CAD build for the part. Positions are in the model's coordinates, mm. Face numbers are marked on the shaded views. A direction names the side the tool comes from. Give positions to 0.01 mm unless a question says otherwise; leave off trailing zeros. Loops run counter-clockwise (first coordinate to the right, second up) from the corner with the lowest first, then second, coordinate; pieces in that order, holes last. Notation, with made-up numbers: M 50.5,41.25 L 99.5,41.25 A16 ccw 99.5,57.25 Z; hole C 53.5,16 d2. An arc over 180 degrees is marked long. Answer as CSV lines item,"result".
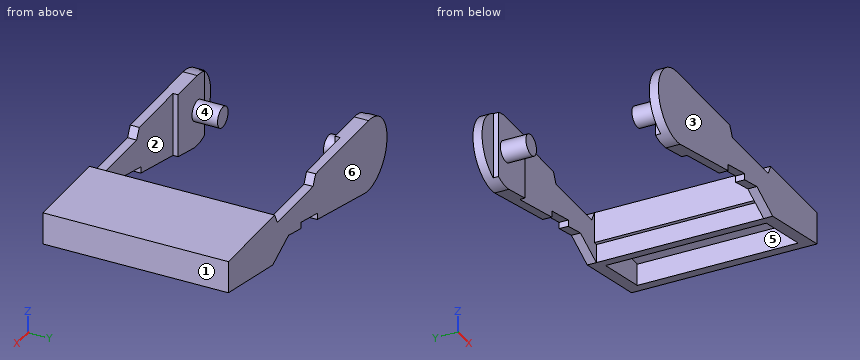
from build123d import *

# Parameters (mm, degrees)
CYLINDER_R        = 0.8
CYLINDER_DEPTH    = 2
CYLINDER001_R     = 0.8
CYLINDER001_DEPTH = 2
BOX004_W          = 0.3
BOX004_H          = 12.95
BOX004_DEPTH      = 3.2
BOX003_W          = 4.8
BOX003_H          = 12.45
BOX003_DEPTH      = 4.6
BOX001_W          = 1.7
BOX001_H          = 12.95
BOX001_DEPTH      = 10
BOX002_W          = 11.3
BOX002_H          = 12.95
BOX002_DEPTH      = 10
BOX_W             = 15.8
BOX_H             = 12.15
BOX_DEPTH         = 10
EXTRUDE_DEPTH     = 14.35


with BuildPart() as cylinder:
    # Cylinder → Cylinder (new body)
    with BuildSketch(Plane(origin=(2.8, -4.1, 2.8), x_dir=(1, 0, 0), z_dir=(0, -1, 0))):
        Circle(CYLINDER_R)
    extrude(amount=CYLINDER_DEPTH)


with BuildPart() as cylinder001:
    # Cylinder001 → Cylinder001 (new body)
    with BuildSketch(Plane(origin=(2.8, 6.1, 2.8), x_dir=(1, 0, 0), z_dir=(0, -1, 0))):
        Circle(CYLINDER001_R)
    extrude(amount=CYLINDER001_DEPTH)


with BuildPart() as cube004:
    # Box004 → Box004 (new body)
    with BuildSketch(Plane(origin=(17, -6.475, 0), x_dir=(1, 0, 0), z_dir=(0, 0, 1))):
        with Locations((0.15, 6.475)):
            Rectangle(BOX004_W, BOX004_H)
    extrude(amount=BOX004_DEPTH)


with BuildPart() as compound001:
    # Box003 → Box003 (new body)
    with BuildSketch(Plane(origin=(18.2, -6.225, 0), x_dir=(1, 0, 0), z_dir=(0, 0, 1))):
        with Locations((2.4, 6.225)):
            Rectangle(BOX003_W, BOX003_H)
    extrude(amount=BOX003_DEPTH)

    # Compound001: union Cube004
    add(cube004.part)


with BuildPart() as cube001:
    # Box001 → Box001 (new body)
    with BuildSketch(Plane(origin=(0, -6.475, 0), x_dir=(1, 0, 0), z_dir=(0, 0, 1))):
        with Locations((0.85, 6.475)):
            Rectangle(BOX001_W, BOX001_H)
    extrude(amount=BOX001_DEPTH)


with BuildPart() as compound:
    # Box002 → Box002 (new body)
    with BuildSketch(Plane(origin=(5.7, -6.475, 0), x_dir=(1, 0, 0), z_dir=(0, 0, 1))):
        with Locations((5.65, 6.475)):
            Rectangle(BOX002_W, BOX002_H)
    extrude(amount=BOX002_DEPTH)

    # Compound: union Cube001
    add(cube001.part)


with BuildPart() as cube:
    # Box → Box (new body)
    with BuildSketch(Plane(origin=(0, -6.075, 0), x_dir=(1, 0, 0), z_dir=(0, 0, 1))):
        with Locations((7.9, 6.075)):
            Rectangle(BOX_W, BOX_H)
    extrude(amount=BOX_DEPTH)


with BuildPart() as fusion:
    # Sketch → Extrude (new body)
    with BuildSketch(Plane.XZ):
        with BuildLine():
            ThreePointArc((2.8, 5.6), (0.010655, 2.555964), (3.286215, 0.042538))
            Line((3.286215, 0.042538), (10.556406, 1.8))
            Line((10.556406, 1.8), (10.556406, 2.3))
            Line((10.556406, 2.3), (13.056406, 2.904338))
            Line((13.056406, 2.404338), (13.056406, 2.904338))
            Line((13.056406, 2.404338), (14.9, 2.85))
            Line((14.9, 2.85), (17.3, 1.75))
            Line((17.3, 1.75), (24, 3.1))
            Line((24, 5.6), (24, 3.1))
            Line((17, 5.6), (24, 5.6))
            Line((16.6, 4.8), (17, 5.6))
            Line((11.2, 4.8), (16.6, 4.8))
            Line((11.2, 4.8), (10.8, 5.6))
            Line((2.8, 5.6), (10.8, 5.6))
        make_face()
    extrude(amount=EXTRUDE_DEPTH)


with BuildPart() as fusion_1:
    # Extrude placement: moved
    add(fusion.part.moved(Location((0, 7.175, 0))))

    # Cut: cut Cube
    add(cube.part, mode=Mode.SUBTRACT)

    # Cut001: cut Compound
    add(compound.part, mode=Mode.SUBTRACT)

    # Cut002: cut Compound001
    add(compound001.part, mode=Mode.SUBTRACT)

    # Fusion: union Cylinder, Cylinder001
    add(cylinder.part)
    add(cylinder001.part)


solid = fusion_1.part
1) Which spindle directions (+Z, -Z, +X, -X, +Y, -Y) get a long thin tool onto all of the face, cutting with end or side? Do the marked faces 4, 5 and 6. Say none if no direction does.
Answer below:
face 4,"none"
face 5,"-Z"
face 6,"+Z, -Z, +X, -X, +Y"
2) Drill centre lines: line 1 (Y direction, x = 14.25, z = 3.4) (3 decimals); line 2 (Y direction, x = 18.25, z = 3.95) (3 decimals); line 3 (X direction, y = 4.5, z = 4.2). Where is each one in solid material? Low to high. Write a range as from..to.
Answer below:
line 1,"y = -7.175..-6.475, 6.475..7.175"
line 2,"y = -7.175..-6.225, 6.225..7.175"
line 3,"x = 17..18.2, 23..24"
3) Flat gauge pins, fed straight in: pin 1 (1.5 mm diameter, centred on x = 18, y = 1.5, fed in from -Z); pin 2 (0.8 mm diameter, centred on x = 13, y = 7, fed in from +Z); pin 3 (4 mm diameter, centred on x = 20.5, y = 3, fed in from -Z). Where does each tip first touch, or does it go through?
Answer below:
pin 1,"stops at z = 1.75"
pin 2,"stops at z = 4.8"
pin 3,"stops at z = 4.6"
4) Band-saw the part on A-A on y = 3.5. Give the cut face in (x, z).
Answer below:
outline,"M 17,3.2 L 17.3,3.2 L 17.3,1.75 L 18.2,1.93 L 18.2,4.6 L 23,4.6 L 23,2.9 L 24,3.1 L 24,5.6 L 17,5.6 Z"
5) Band-saw the part on B-B on x = 5.25. Give the cut face in (y, z) (3 decimals), and give its area (3 significant figures).
Answer below:
outline,"M -7.175,0.517 L -6.075,0.517 L -6.075,5.6 L -7.175,5.6 Z; M 6.075,0.517 L 7.175,0.517 L 7.175,5.6 L 6.075,5.6 Z"
area,"11.2 mm^2"
6) Mould opens along X. For the marked faces 1, 2 and 3 say: +X half, -X half, draft (parallel to the pull), parting line (faces both ways), or undercut.
Answer below:
face 1,"+X half"
face 2,"undercut"
face 3,"draft"
7) Band-saw the part on D-D on x = 9.75. Give the cut face in (y, z) (3 decimals).
Answer below:
outline,"M -7.175,1.605 L -6.475,1.605 L -6.475,5.6 L -7.175,5.6 Z; M 6.475,1.605 L 7.175,1.605 L 7.175,5.6 L 6.475,5.6 Z"
8) Band-saw the part on C-C on x = 20.5. Give the cut face in (y, z) (3 decimals).
Answer below:
outline,"M -7.175,2.395 L -6.225,2.395 L -6.225,4.6 L 6.225,4.6 L 6.225,2.395 L 7.175,2.395 L 7.175,5.6 L -7.175,5.6 Z"
